Can you work these out from the drawing? Everything is in mm from the part's minimum corner. A direction names the side the tool comes from. Coordinates: 2 decimals unless noted, no trailing zeros. Order: outer loops, then holes, each group sorted by start corner. A loop starts at its lowest first (then second) coordinate and runs counter-clockwise, first axis right, second up. Notation, with made-up numbers: (-25, -16.5) - (-8, -16.5) arc R22 cw to (-8, 22.5) - close; hole circle Ø1 at (71.25, -8). An arc over 180 degrees is marked (long way). One line per item, written item: value.
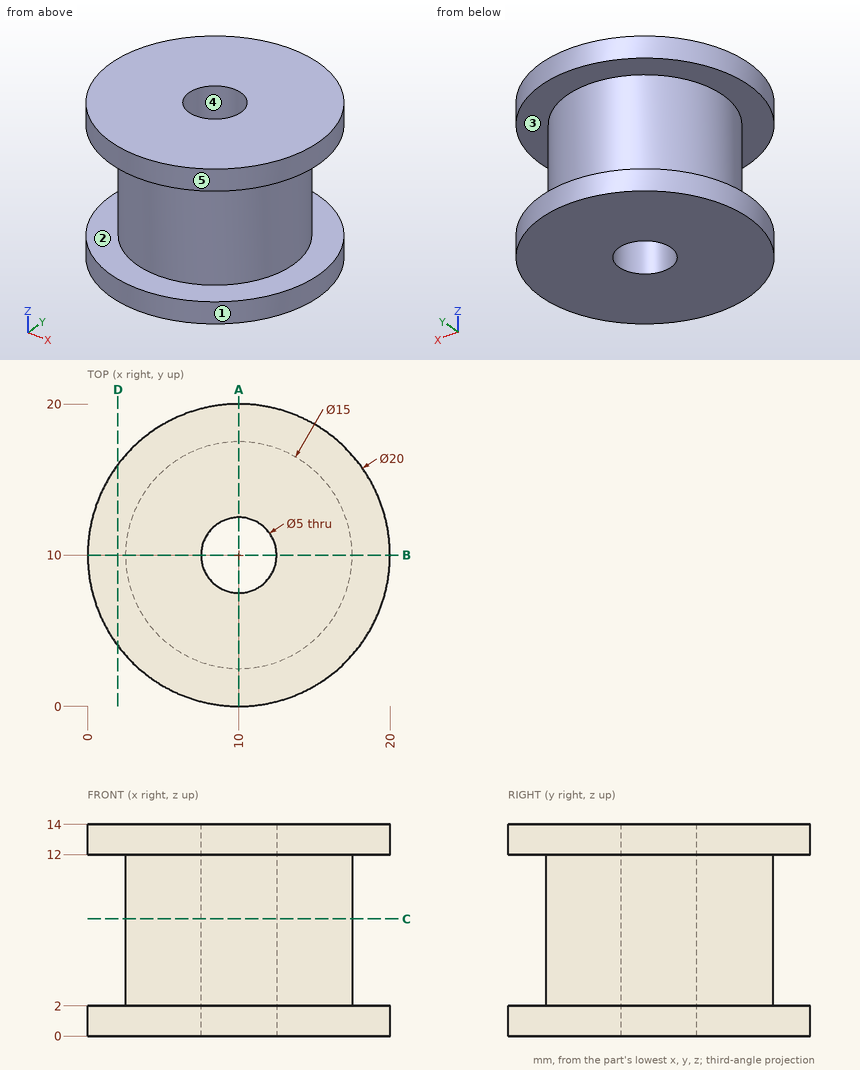
Item 1: I want a section at C-C on z = 7.75. Please give me the cut outline in (x, y), then the cut area to 3 significant figures.
Conclusion:
outline: circle Ø15 at (10, 10); hole circle Ø5 at (10, 10)
area: 157 mm²
Item 2: If I drill on probe 1 along Y at (x, z) = (10, 3.5); probe 2 along Z at (x, y) = (2, 14); probe 3 along Y at (x, z) = (8.25, 1.5), over which ranges is the centre line in solid material (lowest first)?
Conclusion:
probe 1: 2.5 to 7.5, 12.5 to 17.5
probe 2: 0 to 2, 12 to 14
probe 3: 0.15 to 8.21, 11.79 to 19.85
Item 3: Thinking about a two-plate mould opening in Y: for the marked faces 3, 4 and 5, which applies, pulls with the +Y half, pulls with the -Y half, needs draft (parallel to the pull), parting line crosses it, or undercut?
Conclusion:
face 3: needs draft
face 4: undercut
face 5: parting line crosses it
Item 4: I want a section at D-D on x = 2. Please give me the cut outline in (y, z).
Conclusion:
outline: (4, 0) - (16, 0) - (16, 2) - (4, 2) - close; (4, 12) - (16, 12) - (16, 14) - (4, 14) - close
Item 5: For the marked faces 1 and 2, which set-ups out of +Z, -Z, +X, -X, +Y, -Y let a thin tool reach every point of the face, with its end or its side?
Conclusion:
face 1: +Z, -Z
face 2: none
Item 6: I want a section at A-A on x = 10. Please give me the cut outline in (y, z).
Conclusion:
outline: (0, 0) - (7.5, 0) - (7.5, 14) - (0, 14) - (0, 12) - (2.5, 12) - (2.5, 2) - (0, 2) - close; (12.5, 0) - (20, 0) - (20, 2) - (17.5, 2) - (17.5, 12) - (20, 12) - (20, 14) - (12.5, 14) - close
Item 7: I'm going to push flat-ended pins straight in: pin 1 Ø3 at (y, z) = (5, 6.5) entering from -X; pin 2 Ø1 at (y, z) = (3, 10.5) entering from +X; pin 3 Ø6 at (y, z) = (17, 2) entering from -X. Where does each tip first touch, or does it pass through?
Conclusion:
pin 1: x = 3.37
pin 2: x = 13.74
pin 3: x = 0.83
